Work out the finished part from the listing and answer in its coordinate system (mm). A direction names the side the tool comes from. Round coordinates to 2 decimals unless told otherwise and drop trailing zeros. Order: outer loops, then holes, each group sorted by start corner. A loop starts at its lowest first (then second) coordinate and runs counter-clockwise, first axis right, second up. Notation, with made-up numbers: (70.25, 88.25) - (110.25, 88.25) arc R23 cw to (110.25, 127.25) - close; hole circle Ø9 at (35.5, 84). An arc over 180 degrees is marked (long way). One line per question, with ' | ' between items. Start each with the question number.
from build123d import *
from build123d.topology import SkipClean

# Parameters (mm, degrees)
SKETCH1_R           = 88.9
SKETCH1_R_2         = 14.224
BOSS_EXTRUDE1_DEPTH = 3.81
SKETCH3_R           = 38.1
SKETCH3_R_2         = 35.56
BOSS_EXTRUDE3_DEPTH = 7.62
BOSS_EXTRUDE4_DEPTH = 7.62
SKETCH4_R           = 16
SKETCH4_R_2         = 11
BOSS_EXTRUDE5_DEPTH = 7


with BuildPart() as part:
    # Sketch1 → Boss-Extrude1 (new body)
    with BuildSketch(Plane(origin=(0, 0, 0), x_dir=(1, 0, 0), z_dir=(0, 1, 0))):
        with Locations(Location((0, 0, 0), (0, 0, 90))):
            Circle(SKETCH1_R)
        with Locations(Location((-69.85, 0, 0), (0, 0, 90))):
            Circle(SKETCH1_R_2, mode=Mode.SUBTRACT)
        with Locations(Location((-60.491874454, 34.925, 0), (0, 0, 90))):
            Circle(SKETCH1_R_2, mode=Mode.SUBTRACT)
        with Locations(Location((-34.925, 60.491874454, 0), (0, 0, 90))):
            Circle(SKETCH1_R_2, mode=Mode.SUBTRACT)
        with Locations(Location((0, 69.85, 0), (0, 0, 90))):
            Circle(SKETCH1_R_2, mode=Mode.SUBTRACT)
        with Locations(Location((34.925, 60.491874454, 0), (0, 0, 90))):
            Circle(SKETCH1_R_2, mode=Mode.SUBTRACT)
        with Locations(Location((60.491874454, 34.925, 0), (0, 0, 90))):
            Circle(SKETCH1_R_2, mode=Mode.SUBTRACT)
        with Locations(Location((69.85, 0, 0), (0, 0, 90))):
            Circle(SKETCH1_R_2, mode=Mode.SUBTRACT)
        with Locations(Location((60.491874454, -34.925, 0), (0, 0, 90))):
            Circle(SKETCH1_R_2, mode=Mode.SUBTRACT)
        with Locations(Location((34.925, -60.491874454, 0), (0, 0, 90))):
            Circle(SKETCH1_R_2, mode=Mode.SUBTRACT)
    extrude(amount=BOSS_EXTRUDE1_DEPTH)

    # Sketch3 → Boss-Extrude3 (add)
    with BuildSketch(Plane(origin=(0, 3.81, 0), x_dir=(1, 0, 0), z_dir=(0, 1, 0))):
        with Locations(Location((0, 0, 0), (0, 0, 90))):
            Circle(SKETCH3_R)
        with Locations(Location((0, 0, 0), (0, 0, 90))):
            Circle(SKETCH3_R_2, mode=Mode.SUBTRACT)
    extrude(amount=BOSS_EXTRUDE3_DEPTH)

    # Sketch2 → Boss-Extrude4 (add)
    with SkipClean():  # the faces are left unmerged after this step: merging them gives an invalid solid
        with BuildSketch(Plane(origin=(0, 3.81, 0), x_dir=(1, 0, 0), z_dir=(0, 1, 0))):
            with BuildLine():
                Line((-86.19074337, -21.779939332), (-37.110023056, -8.62879996))
                ThreePointArc((-37.110023056, -8.62879996), (-36.801773982, -9.861005618), (-36.452622682, -11.082251559))
                Line((-36.452622682, -11.082251559), (-85.533342996, -24.233390931))
                ThreePointArc((-85.533342996, -24.233390931), (-85.870805957, -23.00901311), (-86.19074337, -21.779939332))
            make_face()
            with BuildLine():
                Line((-85.533342996, 24.233390931), (-36.452622682, 11.082251559))
                ThreePointArc((-36.452622682, 11.082251559), (-36.801773982, 9.861005618), (-37.110023056, 8.62879996))
                Line((-37.110023056, 8.62879996), (-86.19074337, 21.779939332))
                ThreePointArc((-86.19074337, 21.779939332), (-85.870805957, 23.00901311), (-85.533342996, 24.233390931))
            make_face()
            with BuildLine():
                Line((-61.957352439, 63.753403664), (-26.027771498, 27.823822722))
                ThreePointArc((-26.027771498, 27.823822722), (-26.940768363, 26.940768363), (-27.823822722, 26.027771498))
                Line((-27.823822722, 26.027771498), (-63.753403664, 61.957352439))
                ThreePointArc((-63.753403664, 61.957352439), (-62.861792847, 62.861792847), (-61.957352439, 63.753403664))
            make_face()
            with BuildLine():
                Line((-21.779939332, 86.19074337), (-8.62879996, 37.110023056))
                ThreePointArc((-8.62879996, 37.110023056), (-9.861005618, 36.801773982), (-11.082251559, 36.452622682))
                Line((-11.082251559, 36.452622682), (-24.233390931, 85.533342996))
                ThreePointArc((-24.233390931, 85.533342996), (-23.00901311, 85.870805957), (-21.779939332, 86.19074337))
            make_face()
            with BuildLine():
                Line((24.233390931, 85.533342996), (11.082251559, 36.452622682))
                ThreePointArc((11.082251559, 36.452622682), (9.861005618, 36.801773982), (8.62879996, 37.110023056))
                Line((8.62879996, 37.110023056), (21.779939332, 86.19074337))
                ThreePointArc((21.779939332, 86.19074337), (23.00901311, 85.870805957), (24.233390931, 85.533342996))
            make_face()
            with BuildLine():
                Line((63.753403664, 61.957352439), (27.823822722, 26.027771498))
                ThreePointArc((27.823822722, 26.027771498), (26.940768363, 26.940768363), (26.027771498, 27.823822722))
                Line((26.027771498, 27.823822722), (61.957352439, 63.753403664))
                ThreePointArc((61.957352439, 63.753403664), (62.861792847, 62.861792847), (63.753403664, 61.957352439))
            make_face()
            with BuildLine():
                Line((86.19074337, 21.779939332), (37.110023056, 8.62879996))
                ThreePointArc((37.110023056, 8.62879996), (36.801773982, 9.861005618), (36.452622682, 11.082251559))
                Line((36.452622682, 11.082251559), (85.533342996, 24.233390931))
                ThreePointArc((85.533342996, 24.233390931), (85.870805957, 23.00901311), (86.19074337, 21.779939332))
            make_face()
            with BuildLine():
                Line((85.533342996, -24.233390931), (36.452622682, -11.082251559))
                ThreePointArc((36.452622682, -11.082251559), (36.801773982, -9.861005618), (37.110023056, -8.62879996))
                Line((37.110023056, -8.62879996), (86.19074337, -21.779939332))
                ThreePointArc((86.19074337, -21.779939332), (85.870805957, -23.00901311), (85.533342996, -24.233390931))
            make_face()
            with BuildLine():
                Line((61.957352439, -63.753403664), (26.027771498, -27.823822722))
                ThreePointArc((26.027771498, -27.823822722), (26.940768363, -26.940768363), (27.823822722, -26.027771498))
                Line((27.823822722, -26.027771498), (63.753403664, -61.957352439))
                ThreePointArc((63.753403664, -61.957352439), (62.861792847, -62.861792847), (61.957352439, -63.753403664))
            make_face()
            with BuildLine():
                Line((21.779939332, -86.19074337), (8.62879996, -37.110023056))
                ThreePointArc((8.62879996, -37.110023056), (9.861005618, -36.801773982), (11.082251559, -36.452622682))
                Line((11.082251559, -36.452622682), (24.233390931, -85.533342996))
                ThreePointArc((24.233390931, -85.533342996), (23.00901311, -85.870805957), (21.779939332, -86.19074337))
            make_face()
        extrude(amount=BOSS_EXTRUDE4_DEPTH)

    # Sketch4 → Boss-Extrude5 (add)
    with SkipClean():  # the faces are left unmerged after this step: merging them gives an invalid solid
        with BuildSketch(Plane(origin=(0, 3.81, 0), x_dir=(1, 0, 0), z_dir=(0, 1, 0))):
            with Locations(Location((0, 0, 0), (0, 0, 270))):
                Circle(SKETCH4_R)
            with Locations(Location((0, 0, 0), (0, 0, 270))):
                Circle(SKETCH4_R_2, mode=Mode.SUBTRACT)
        extrude(amount=BOSS_EXTRUDE5_DEPTH)


solid = part.part
1) Section B-B on x = 0 is taken. Give the vertices of the cut face in (y, z), and give its area (3 significant figures).
2) Section D-D on x = 69.85 is taken. Give the vertices of the cut face in (y, z).
3) Section C-C on y = 8.75 is taken. Give the number of separate pieces and of enclosed holes in the cut face, and give its area (3 significant figures).
4) Flat-ended cylindrical pins translate along their axes: pin 1 (8 mm diameter, centred on x = -12.5, z = 68.5, fed in from -Y); pin 2 (5 mm diameter, centred on y = 2.5, z = 44.5, fed in from +X); pin 3 (3 mm diameter, centred on y = 5, z = -29.5, fed in from -X); pin 4 (1 mm diameter, centred on y = 3.5, z = 63.5, fed in from -X). Find the tip coordinate at first contact, or state that the pin passes through.
5) Straight lines are drawn through the part: line 1 (X direction, y = 6, z = 0); line 2 (Z direction, x = 69.85, y = 2.85); line 3 (X direction, y = 8.25, z = -28). For each, find the intervals that lie inside material, in ascending order.
6) Determine the mould class of faces 1 (the flat face through (-15.3, 7.6, -62)), 2 (the flat face through (46.04, 7.567, -44.244)), 3 (the flat face through (9, 3.81, -57)) for opening direction Z: released by +Z, released by -Z, zero draft, split by the parting line, or undercut.
7) Section A-A on z = 0 is taken. Give the vertices of the cut face in (x, y), and give its area (3 significant figures).
8) For faces 4 (the flat face through (50, 3.81, -25)), 5 (the flat face through (-62, 7.6, 15.3)), 6 (the flat face through (-44.244, 7.567, -46.04)), determine the directions among +Z, -Z, +X, -X, +Y, -Y from which every point of the face is accessible in a straight line to the end or side of a thin tool.
Recorded:
1) outline: (0, -88.9) - (3.81, -88.9) - (3.81, -84.07) - (0, -84.07) - close; (0, -55.63) - (3.81, -55.63) - (3.81, -38.1) - (11.43, -38.1) - (11.43, -35.56) - (3.81, -35.56) - (3.81, -16) - (10.81, -16) - (10.81, -11) - (3.81, -11) - (3.81, 11) - (10.81, 11) - (10.81, 16) - (3.81, 16) - (3.81, 35.56) - (11.43, 35.56) - (11.43, 38.1) - (3.81, 38.1) - (3.81, 88.9) - (0, 88.9) - close | area: 678 mm²
2) outline: (0, -54.99) - (3.81, -54.99) - (3.81, -45.64) - (0, -45.64) - close; (0, -24.21) - (3.81, -24.21) - (3.81, -20.03) - (11.43, -20.03) - (11.43, -17.4) - (3.81, -17.4) - (3.81, -14.22) - (0, -14.22) - close; (0, 14.22) - (3.81, 14.22) - (3.81, 17.4) - (11.43, 17.4) - (11.43, 20.03) - (3.81, 20.03) - (3.81, 24.21) - (0, 24.21) - close; (0, 45.64) - (3.81, 45.64) - (3.81, 54.99) - (0, 54.99) - close
3) separate pieces: 2 | enclosed holes: 2 | area: 2,300 mm²
4) pin 1: stops at y = 0 | pin 2: stops at x = 78.35 | pin 3: stops at x = -84.18 | pin 4: stops at x = -62.72
5) line 1: x = -38.1 to -35.56, -16 to -11, 11 to 16, 35.56 to 38.1 | line 2: z = -54.99 to -45.64, -24.21 to -14.22, 14.22 to 24.21, 45.64 to 54.99 | line 3: x = -29.8 to -26.2, -25.84 to -21.92, 21.92 to 25.84, 26.2 to 29.8
6) face 1: released by -Z | face 2: undercut | face 3: zero draft
7) outline: (-88.9, 0) - (-84.07, 0) - (-84.07, 3.81) - (-88.9, 3.81) - close; (-55.63, 0) - (55.63, 0) - (55.63, 3.81) - (38.1, 3.81) - (38.1, 11.43) - (35.56, 11.43) - (35.56, 3.81) - (16, 3.81) - (16, 10.81) - (11, 10.81) - (11, 3.81) - (-11, 3.81) - (-11, 10.81) - (-16, 10.81) - (-16, 3.81) - (-35.56, 3.81) - (-35.56, 11.43) - (-38.1, 11.43) - (-38.1, 3.81) - (-55.63, 3.81) - close; (84.07, 0) - (88.9, 0) - (88.9, 3.81) - (84.07, 3.81) - close | area: 569 mm²
8) face 4: +Y | face 5: -X, +Y | face 6: -Z, +Y
